```python
from build123d import *

# Parameters (mm, degrees)
DIGITIZER_DEPTH                               = 2.25
SKETCH2_W                                     = 315
SKETCH2_H                                     = 104
DISPLAY_INCLUDING_ADHESIVE_MARGIN_OF_5M_DEPTH = 2.5
SKETCH3_W                                     = 70
SKETCH3_H                                     = 2.5
DIGITIZER_CABLE_DEPTH                         = 2.5


with BuildPart() as part:
    # Sketch1 → DIGITIZER (new body)
    with BuildSketch(Plane.XY):
        with BuildLine():
            Line((-158, -54.5), (158, -54.5))
            ThreePointArc((158, -54.5), (159.767766953, -53.767766953), (160.5, -52))
            Line((160.5, -52), (160.5, 52))
            ThreePointArc((160.5, 52), (159.767766953, 53.767766953), (158, 54.5))
            Line((158, 54.5), (-158, 54.5))
            ThreePointArc((-158, 54.5), (-159.767766953, 53.767766953), (-160.5, 52))
            Line((-160.5, 52), (-160.5, -52))
            ThreePointArc((-160.5, -52), (-159.767766953, -53.767766953), (-158, -54.5))
        make_face()
    extrude(amount=DIGITIZER_DEPTH)

    # Sketch2 → DISPLAY INCLUDING ADHESIVE MARGIN OF .5MM (add)
    with BuildSketch(Plane(origin=(0, 0, 0), x_dir=(-1, 0, 0), z_dir=(0, 0, -1))):
        Rectangle(SKETCH2_W, SKETCH2_H)
    extrude(amount=DISPLAY_INCLUDING_ADHESIVE_MARGIN_OF_5M_DEPTH)

    # Sketch3 → DIGITIZER CABLE (add)
    with BuildSketch(Plane(origin=(0, 0, 0), x_dir=(-1, 0, 0), z_dir=(0, 0, -1))):
        with Locations((0, -53.25)):
            Rectangle(SKETCH3_W, SKETCH3_H)
    extrude(amount=DIGITIZER_CABLE_DEPTH)


solid = part.part
```
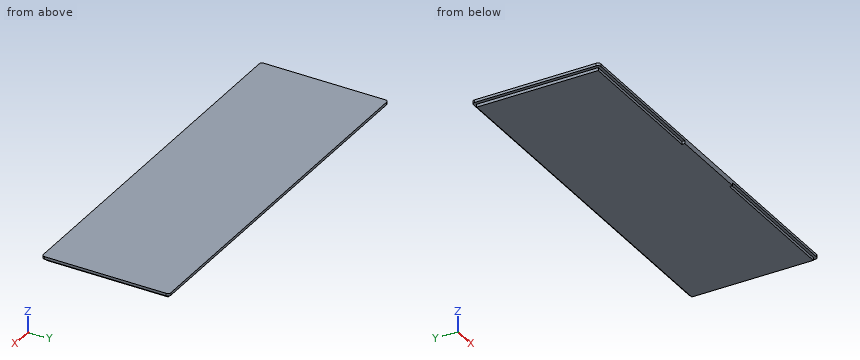
Can you work these out from the model? Positions are in its coordinate system, mm. Coordinates: 2 decimals unless noted, no trailing zeros. Order: outer loops, then holes, each group sorted by start corner. A loop starts at its lowest first (then second) coordinate and runs counter-clockwise, first axis right, second up. Notation, with made-up numbers: (-11.5, 51.5) - (39.5, 51.5) arc R16 ccw to (39.5, 75.5) - close; hole circle Ø5 at (-27.5, 8.5). An arc over 180 degrees is marked (long way). Answer in a Markdown table with one row per item.
1. Suppose I cut it at A-A (z = -0.85). Please give me the cut outline in (x, y).
Reply:
| item | result |
|---|---|
| outline | (-157.5, -52) - (-35, -52) - (-35, -54.5) - (35, -54.5) - (35, -52) - (157.5, -52) - (157.5, 52) - (-157.5, 52) - close |
2. If I drill on line 1 along Y through (x, z) = (-106, -1.95); line 2 along X through (y, z) = (27, -0.5); line 3 along Y through (x, z) = (-33, -0.4), over which ranges is the centre line in solid material (lowest first)?
Reply:
| item | result |
|---|---|
| line 1 | y = -52 to 52 |
| line 2 | x = -157.5 to 157.5 |
| line 3 | y = -54.5 to 52 |
3. For pin 1 (0.8 mm diameter, centred on x = 58.5, z = -1.5, fed in from +Y); pin 2 (0.8 mm diameter, centred on y = 23.5, z = -1, fed in from -X); pin 3 (2 mm diameter, centred on y = 17.5, z = -2, fed in from +X), each with a flat end and sliding along its axis, tell me the tip position at first contact or that it passes through.
Reply:
| item | result |
|---|---|
| pin 1 | stops at y = 52 |
| pin 2 | stops at x = -157.5 |
| pin 3 | stops at x = 157.5 |
4. Suppose I cut it at B-B (x = 106). Please give me the cut outline in (y, z), and give its area (3 significant figures).
Reply:
| item | result |
|---|---|
| outline | (-54.5, 0) - (-52, 0) - (-52, -2.5) - (52, -2.5) - (52, 0) - (54.5, 0) - (54.5, 2.25) - (-54.5, 2.25) - close |
| area | 505 mm^2 |
